Build history of the part. All positions in model axes, mm. A direction names the side the tool comes from. Give positions to 0.01 mm unless a question says otherwise; leave off trailing zeros. Order: outer loops, then holes, each group sorted by start corner. A loop starts at its lowest first (then second) coordinate and runs counter-clockwise, first axis right, second up. Notation, with made-up numbers: (-31.5, -31) - (10.5, -31) arc R30 ccw to (10.5, -9) - close; hole circle Ø1 at (-1, 20). An arc over 180 degrees is marked (long way). Answer in a Markdown table with one row per item.
Autodesk Inventor part; units mm, degrees
ref_plane "YZ Plane" through (0, 0, 0) normal (1, 0, 0) x (0, 1, 0)
ref_plane "XZ Plane" through (0, 0, 0) normal (0, 1, 0) x (-1, 0, 0)
ref_plane "XY Plane" through (0, 0, 0) normal (0, 0, 1) x (1, 0, 0)
sketch "スケッチ2" plane through (0, 0, 0) normal (0, 0, 1) x (1, 0, 0)
  line L0 (0, -106.3056) -> (0, 106.3056)
  line L1 (-64.6, 0) -> (212.6, 0)
  arc A0 (140.9062, 3) -> (140.9062, -3) centre (93, 0) ccw
  line L2 (-25, -25) -> (25, -25)
  line L3 (25, 25) -> (-25, 25)
  line L4 (-25, -25) -> (25, 25) construction
  line L5 (25, -25) -> (-25, 25) construction
  line L6 (25, 25) -> (29.7624, 25)
  line L7 (25, -25) -> (29.7624, -25)
  line L8 (140.9062, -3) -> (173, -3)
  line L9 (173, 3) -> (140.9062, 3)
  line L10 (145.3369, -0.7898) -> (173, 3) construction
  line L11 (173, -3) -> (145.3176, 0.7925) construction
  arc A1 (29.7624, -25) -> (160.5278, -8) centre (93, 0) ccw
  arc A2 (160.5278, 8) -> (29.7624, 25) centre (93, 0) ccw
  line L12 (173, 3) -> (173, 8)
  line L13 (173, 8) -> (160.5278, 8)
  line L14 (173, -3) -> (173, -8)
  line L15 (173, -8) -> (160.5278, -8)
  line L16 (-25, 25) -> (-25, -25)
  point P0 (0, 0)
  point P1 (151.102, 0)
  dimension "d1" = 96
  dimension "d2" = 50
  dimension "d7" = 5
  dimension "d8" = 3
  dimension "d9" = 5
  dimension "d10" = 80
  dimension "d12" = 20
  dimension "d13" = 93
  dimension "d15" = 20
  dimension "d16" = 50
  dimension "d17" = 3
  dimension "d18" = 50
extrude "押し出し1" add sketch "スケッチ2" along normal blind 6
sketch "スケッチ3" plane through (0, 0, 6) normal (0, 0, 1) x (1, 0, 0)
  line L0 (15, -15) -> (-15, -15)
  line L1 (-15, -15) -> (-15, 15)
  line L2 (-15, 15) -> (15, 15)
  line L3 (15, 15) -> (15, -15)
  line L4 (15, -15) -> (-15, 15) construction
  line L5 (-15, -15) -> (15, 15) construction
  circle A0 centre (-15, -15) radius 2.5
  circle A1 centre (-15, 15) radius 2.5
  line L6 (-15, 15) -> (-15, 45)
  circle A2 centre (15, -15) radius 2.5
  circle A3 centre (15, 15) radius 2.5
  point P0 (0, 0)
  dimension "d21" = 30
  dimension "d22" = 30
  dimension "d23" = 5
  dimension "d26" = 30
  dimension "d33" = 30
extrude "押し出し2" cut sketch "スケッチ3" against normal blind 6 contours A0 L1 L0 | L0 L1 A0 | A2 L3 L0 | L0 L3 A2 | A1 L6 L1 | L1 L2 A1 | A3 L2 L3 | L3 L2 A3 | L6 A1 L2
sketch "スケッチ4" plane through (160.5278, -8, 0) normal (0, -1, 0) x (1, 0, 0)
  circle A0 centre (7.4722, 3) radius 2
  line L0 (0, 0) -> (12.4722, 0)
  line L1 (12.4722, 0) -> (12.4722, 6)
  point P0 (-160.5278, 0)
  dimension "d40" = 3
  dimension "d41" = 4
  dimension "d42" = 5
extrude "押し出し3" cut sketch "スケッチ4" against normal through all
properties part number "motor_hold_sample" material "アルミニウム 6061"
1. Which spindle directions (+Z, -Z, +X, -X, +Y, -Y) get a long thin tool onto all of the face, cutting with end or side? Do faces 5 (the face through (165, -8, 3)), 6 (the face through (165, 8, 3)), 7 (the face through (2, -25, 3)), 8 (the face through (157, -3, 3)). Say none if no direction does.
Check result:
| item | result |
|---|---|
| face 5 | +Z, -Z, +X, -Y |
| face 6 | +Z, -Z, +X, +Y |
| face 7 | +Z, -Z, -X, -Y |
| face 8 | +Z, -Z, +X |
2. Cut at D-D on y = -15. Write the cut outline in (x, z).
Check result:
| item | result |
|---|---|
| outline | (-25, 0) - (-17.5, 0) - (-17.5, 6) - (-25, 6) - close; (-12.5, 0) - (12.5, 0) - (12.5, 6) - (-12.5, 6) - close; (17.5, 0) - (47.4, 0) - (47.4, 6) - (17.5, 6) - close; (138.6, 0) - (159.32, 0) - (159.32, 6) - (138.6, 6) - close |
3. Cut at B-B on x = -15. Write the cut outline in (y, z), and give its area (3 significant figures).
Check result:
| item | result |
|---|---|
| outline | (-25, 0) - (-17.5, 0) - (-17.5, 6) - (-25, 6) - close; (-12.5, 0) - (12.5, 0) - (12.5, 6) - (-12.5, 6) - close; (17.5, 0) - (25, 0) - (25, 6) - (17.5, 6) - close |
| area | 240 mm² |
4. Cut at C-C on x = 168. Write the cut outline in (y, z), and give its area (3 significant figures).
Check result:
| item | result |
|---|---|
| outline | (-8, 0) - (-3, 0) - (-3, 1) - (-8, 1) - close; (-8, 5) - (-3, 5) - (-3, 6) - (-8, 6) - close; (3, 0) - (8, 0) - (8, 1) - (3, 1) - close; (3, 5) - (8, 5) - (8, 6) - (3, 6) - close |
| area | 20.0 mm² |
5. Drop flat-ended pins along their axis: P1, Ø3, axis at y = -33.5, z = 1, coming from the +X side; P2, Ø1.8, axis at x = 8.5, z = 4, coming from the -Y side; P3, Ø3, axis at y = -45, z = 2.5, coming from the +X side. Give the stop position or say it passes through.
Check result:
| item | result |
|---|---|
| P1 | stops at x = 153 |
| P2 | stops at y = -25 |
| P3 | stops at x = 145.27 |
6. Probe line 1 (Y direction, x = -15, z = 2.8); line 2 (Z direction, x = 168, y = -4); line 3 (Y direction, x = 94.5, z = 1.65). List the from-to ranges inside material, lowest first.
Check result:
| item | result |
|---|---|
| line 1 | y = -25 to -17.5, -12.5 to 12.5, 17.5 to 25 |
| line 2 | z = 0 to 1, 5 to 6 |
| line 3 | y = -67.98 to -47.98, 47.98 to 67.98 |
7. Two-plate mould, pull along X, no slides. Class faces 1 (the face through (-25, 0, 3)), 2 (the face through (166, -6, 3)), 3 (the face through (3, 25, 3)), 4 (the face through (166, 5, 3)): +X half, -X half, draft (parallel to the pull), parting line (faces both ways), or undercut.
Check result:
| item | result |
|---|---|
| face 1 | -X half |
| face 2 | undercut |
| face 3 | draft |
| face 4 | undercut |
8. Cut at A-A on z = 3. Write the cut outline in (x, y).
Check result:
| item | result |
|---|---|
| outline | (-25, -25) - (29.76, -25) arc R68 ccw to (160.53, -8) - (166, -8) - (166, -3) - (140.91, -3) arc R48 cw (long way) to (140.91, 3) - (166, 3) - (166, 8) - (160.53, 8) arc R68 ccw to (29.76, 25) - (-25, 25) - close; (170, -8) - (173, -8) - (173, -3) - (170, -3) - close; (170, 3) - (173, 3) - (173, 8) - (170, 8) - close; hole circle Ø5 at (-15, -15); hole circle Ø5 at (-15, 15); hole circle Ø5 at (15, -15); hole circle Ø5 at (15, 15) |
